Autodesk Inventor part; units mm, degrees
ref_plane "YZ Plane" through (0, 0, 0) normal (1, 0, 0) x (0, 1, 0)
ref_plane "XZ Plane" through (0, 0, 0) normal (0, 1, 0) x (-1, 0, 0)
ref_plane "XY Plane" through (0, 0, 0) normal (0, 0, 1) x (1, 0, 0)
sketch "Boceto1" plane through (0, 0, 0) normal (1, 0, 0) x (0, 1, 0)
  line L0 (0, 64.5) -> (0, -64.5)
  line L1 (2, 64.5) -> (5, 64.5)
  line L2 (5, 64.5) -> (5, -64.5)
  line L3 (5, -64.5) -> (2, -64.5)
  line L4 (2, -64.5) -> (2, 64.5)
  point P0 (0, 0)
  point P1 (0, 0)
  dimension "d0" = 129
  dimension "d1" = 10
  dimension "d3" = 3
revolve "Revolución1" add sketch "Boceto1" angle 360 about axis through (0, 0, 64.5) along (0, 0, -1)
thread "Rosca1"
chamfer "Chaflán1" distance 0.5 angle 45 4 edges at (0, -2, 64.5) (0, -5, 64.5) (0, -5, -64.5) (0, -2, -64.5)
properties part number "eje manzana"
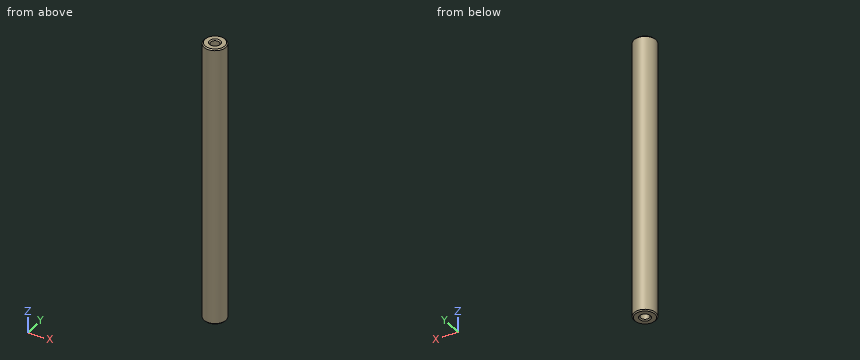
Part model, mm, in its own coordinate system. Coordinates: 2 decimals unless noted, no trailing zeros. Order: outer loops, then holes, each group sorted by start corner. A loop starts at its lowest first (then second) coordinate and runs counter-clockwise, first axis right, second up. Notation, with made-up numbers: M -26.75,14 L 19.25,14 A22 cw 19.25,53 Z; hole C 89,9.25 d1. An arc over 180 degrees is marked long. One line per question, with ' | ' between items.
Q1. Drill centre lines: line 1 (X direction, y = 0, z = 15.5); line 2 (Y direction, x = 0.25, z = 22.5); line 3 (Z direction, x = -4.5, y = -0.25). Where is each one in solid material? Low to high.
A:
line 1: x = -5 to -2, 2 to 5 | line 2: y = -4.99 to -1.98, 1.98 to 4.99 | line 3: z = -64.49 to 64.49
Q2. Slice it at A-A (x = 0). Give the cut face in (y, z).
A:
outline: M -5,-64 L -4.5,-64.5 L -2.5,-64.5 L -2,-64 L -2,64 L -2.5,64.5 L -4.5,64.5 L -5,64 Z; M 2,-64 L 2.5,-64.5 L 4.5,-64.5 L 5,-64 L 5,64 L 4.5,64.5 L 2.5,64.5 L 2,64 Z
Q3. Slice it at C-C (z = 14.5). Give the cut face in (x, y).
A:
outline: C 0,0 d10; hole C 0,0 d4
Q4. Pin check, flat tips, straight feed: P1, Ø3, axis at y = 3.5, z = -6, coming from the +X side; P2, Ø3, axis at x = 1, y = 2, coming from the +Z side; P3, Ø1.5, axis at x = 1, y = 1, coming from the -Z side; P4, Ø4, axis at x = -3.5, z = -25, coming from the -Y side. Stop position of each tip, or through.
A:
P1: stops at x = 4.58 | P2: stops at z = 64.5 | P3: stops at z = -64.16 | P4: stops at y = -4.77
